```python
from build123d import *

# Parameters (mm, degrees)
SKETCH1_W           = 150.368
SKETCH1_H           = 150.368
BOSS_EXTRUDE1_DEPTH = 6.858
SKETCH2_W           = 203.2
SKETCH2_H           = 198.374
BOSS_EXTRUDE2_DEPTH = 6.858
SKETCH5_R           = 2.286
CUT_EXTRUDE2_DEPTH  = 6.858
SKETCH6_W           = 18.288
SKETCH6_H           = 10.16
SKETCH6_W_2         = 24.384
SKETCH6_H_2         = 16.002
CUT_EXTRUDE3_DEPTH  = 6.858
SKETCH8_R           = 2.45030007
SKETCH8_R_2         = 2.286
CUT_EXTRUDE8_DEPTH  = 6.858
CUT_EXTRUDE10_DEPTH = 6.858
SKETCH9_W           = 150.368
SKETCH9_H           = 150.368
CUT_EXTRUDE11_DEPTH = 5.08
SKETCH4_R           = 2.286
CUT_EXTRUDE12_DEPTH = 6.858


with BuildPart() as part:
    # Sketch1 → Boss-Extrude1 (new body)
    with BuildSketch(Plane(origin=(0, 0, 0), x_dir=(1, 0, 0), z_dir=(0, 1, 0))):
        Rectangle(SKETCH1_W, SKETCH1_H)
    extrude(amount=BOSS_EXTRUDE1_DEPTH)

    # Sketch2 → Boss-Extrude2 (add)
    with BuildSketch(Plane(origin=(0, 6.858, 0), x_dir=(1, 0, 0), z_dir=(0, 1, 0))):
        Rectangle(SKETCH2_W, SKETCH2_H)
    extrude(amount=-BOSS_EXTRUDE2_DEPTH)

    # Sketch5 → Cut-Extrude2 (cut)
    with BuildSketch(Plane(origin=(0, 6.858, 0), x_dir=(1, 0, 0), z_dir=(0, 1, 0))):
        with Locations((-8.889186327, -85.126681614)):
            Circle(SKETCH5_R)
        with Locations((8.890813673, -85.126681614)):
            Circle(SKETCH5_R)
    extrude(amount=-CUT_EXTRUDE2_DEPTH, mode=Mode.SUBTRACT)

    # Sketch6 → Cut-Extrude3 (cut)
    with BuildSketch(Plane(origin=(0, 0, 0), x_dir=(-1, 0, 0), z_dir=(0, -1, 0))):
        with Locations((-39.624813673, -87.111607671)):
            Rectangle(SKETCH6_W, SKETCH6_H)
        with Locations((42.671186327, -87.111607671)):
            Rectangle(SKETCH6_W_2, SKETCH6_H_2)
    extrude(amount=-CUT_EXTRUDE3_DEPTH, mode=Mode.SUBTRACT)

    # Sketch8 → Cut-Extrude8 (cut)
    with BuildSketch(Plane(origin=(0, 6.858, 0), x_dir=(1, 0, 0), z_dir=(0, 1, 0))):
        with Locations((-89.861846327, -87.359341614)):
            Circle(SKETCH8_R)
        with Locations((89.863473673, -87.359341614)):
            Circle(SKETCH8_R_2)
        with Locations((89.863473673, 87.539978386)):
            Circle(SKETCH8_R_2)
        with Locations((-89.861846327, 87.448846327)):
            Circle(SKETCH8_R_2)
    extrude(amount=-CUT_EXTRUDE8_DEPTH, mode=Mode.SUBTRACT)

    # Sketch7 → Cut-Extrude10 (cut)
    with BuildSketch(Plane(origin=(0, 6.858, 0), x_dir=(1, 0, 0), z_dir=(0, 1, 0))):
        Polygon((101.6, -99.187), (101.6, -92.747495287), (95.341132059, -99.187), align=None)
        Polygon((-95.339504713, 99.187), (-101.6, 99.187), (-101.6, 93.007109855), align=None)
        Polygon((101.6, 92.928132059), (101.6, 99.187), (95.341132059, 99.187), align=None)
        Polygon((-101.6, -92.747495287), (-95.180018996, -99.187), (-101.6, -99.187), align=None)
    extrude(amount=-CUT_EXTRUDE10_DEPTH, mode=Mode.SUBTRACT)

    # Sketch9 → Cut-Extrude11 (cut)
    with BuildSketch(Plane(origin=(0, 0, 0), x_dir=(-1, 0, 0), z_dir=(0, -1, 0))):
        with Locations((0, 3.700326738)):
            Rectangle(SKETCH9_W, SKETCH9_H)
    extrude(amount=-CUT_EXTRUDE11_DEPTH, mode=Mode.SUBTRACT)

    # Sketch4 → Cut-Extrude12 (cut)
    with BuildSketch(Plane(origin=(0, 6.858, 0), x_dir=(1, 0, 0), z_dir=(0, 1, 0))):
        with Locations((0.000813673, -80.046681614)):
            Circle(SKETCH4_R)
    extrude(amount=-CUT_EXTRUDE12_DEPTH, mode=Mode.SUBTRACT)


solid = part.part
```
CAD build for the part. Positions are in the model's coordinates, mm. A direction names the side the tool comes from. Round coordinates to 2 decimals unless told otherwise and drop trailing zeros. Write each loop counter-clockwise with the first axis right and the second up, starting at its lowest first coordinate (ties: lowest second). Pieces come first, ordered by that corner, then holes. Notation, with made-up numbers: (16.5, 81) -> (60.5, 81) arc R24 ccw to (60.5, 105) -> close; hole circle Ø1 at (89.25, -1). An arc over 180 degrees is marked (long way). Answer in a Markdown table with one row per item. Add a question column.
Item 1: Saw through at C-C, the plane z = -2. Write the cut outline in (x, y).
Item 2: Mould opens along X. For faces 4 (the face through (0, 0, 73)), 5 (the face through (1, 3, -78.884)), 6 (the face through (-98.435, 3.477, 95.922)) say: pulls with the +X half, pulls with the -X half, needs draft (parallel to the pull), parting line crosses it, or undercut.
Item 3: Saw through at D-D, the plane y = 2.75. Count the separate pieces of the cut face and the enclosed holes in it, then the cut area to 3 significant figures.
Item 4: Saw through at A-A, the plane x = -36. Write the cut outline in (y, z).
Item 5: Saw through at B-B, the plane x = -64.5. Write the cut outline in (y, z), then the cut area to 3 significant figures.
Item 6: Drop a flat-ended pin along its axis: pin 1 Ø2.5 at (x, z) = (89.86, -87.54) entering from +Y. Give the stop position or say it passes through.
Item 7: Drill centre lines: line 1 (Z direction, x = 32.5, y = 4); line 2 (X direction, y = 3, z = -6); line 3 (Z direction, x = -47, y = 6.75). Where is each one in solid material? Low to high. Write a range as from..to.
Item 8: Which spindle directions (+Z, -Z, +X, -X, +Y, -Y) get a long thin tool onto all of the face, cutting with end or side? Do faces 1 (the face through (-43, 3, 79.111)), 2 (the face through (-101.6, 3, 1)), 3 (the face through (-75.184, 3, -3)). Say none if no direction does.
Findings below:
| question | item | result |
|---|---|---|
| 1 | outline | (-101.6, 0) -> (-75.18, 0) -> (-75.18, 5.08) -> (75.18, 5.08) -> (75.18, 0) -> (101.6, 0) -> (101.6, 6.86) -> (-101.6, 6.86) -> close |
| 2 | face 4 | needs draft |
| 2 | face 5 | undercut |
| 2 | face 6 | pulls with the -X half |
| 3 | separate pieces | 1 |
| 3 | enclosed holes | 10 |
| 3 | area | 16,900 mm^2 |
| 4 | outline | (0, -99.19) -> (6.86, -99.19) -> (6.86, 79.11) -> (0, 79.11) -> (0, 71.48) -> (5.08, 71.48) -> (5.08, -78.88) -> (0, -78.88) -> close; (0, 95.11) -> (6.86, 95.11) -> (6.86, 99.19) -> (0, 99.19) -> close |
| 5 | outline | (0, -99.19) -> (6.86, -99.19) -> (6.86, 99.19) -> (0, 99.19) -> (0, 71.48) -> (5.08, 71.48) -> (5.08, -78.88) -> (0, -78.88) -> close |
| 5 | area | 597 mm^2 |
| 6 | pin 1 | passes through |
| 7 | line 1 | z = -99.19..-78.88, 71.48..82.03, 92.19..99.19 |
| 7 | line 2 | x = -101.6..-75.18, 75.18..101.6 |
| 7 | line 3 | z = -99.19..79.11, 95.11..99.19 |
| 8 | face 1 | +Y, -Y |
| 8 | face 2 | +Z, -Z, -X, +Y, -Y |
| 8 | face 3 | -Y |
